Input: part model. Units: mm. Frame: model coordinates. A direction names the side the tool comes from. Give positions to 0.01 mm unless a question says otherwise; leave off trailing zeros. Order: outer loops, then holes, each group sorted by start corner. A loop starts at its lowest first (then second) coordinate and runs counter-clockwise, first axis right, second up. Notation, with made-up numbers: M -39,-38 L -8,-38 A36 cw -8,-1 Z; hole C -7,89.25 d1. An arc over 180 degrees is marked long. Use a Markdown table: item, result.
from build123d import *

# Parameters (mm, degrees)
BOSS_EXTRUDE1_DEPTH = 10
SKETCH2_R           = 1.5
CUT_EXTRUDE1_DEPTH  = 30


with BuildPart() as part:
    # Sketch1 → Boss-Extrude1 (new body)
    with BuildSketch(Plane.XY):
        with BuildLine():
            Line((-3, -2), (-14.8, -2))
            Line((-14.8, -2), (-15, -1.8))
            Line((-15, -1.8), (-15, -0.7))
            Line((-15, -0.7), (-14.8, -0.5))
            Line((-14.8, -0.5), (-4.866025404, -0.5))
            ThreePointArc((-4.866025404, -0.5), (-4.366025404, -0.366025404), (-4, 0))
            ThreePointArc((-4, 0), (-2.828427125, 2.828427125), (0, 4))
            Line((0, 4), (0, 2))
            ThreePointArc((0, 2), (-1.414213562, 1.414213562), (-2, 0))
            Line((-2, 0), (-2, -1))
            ThreePointArc((-2, -1), (-2.292893219, -1.707106781), (-3, -2))
        make_face()
    boss_extrude1 = extrude(amount=BOSS_EXTRUDE1_DEPTH)

    # Sketch2 → Cut-Extrude1 (cut)
    with BuildSketch(Plane(origin=(0, -0.5, 0), x_dir=(1, 0, 0), z_dir=(0, 1, 0))):
        with Locations(Location((-10, -5, 0), (0, 0, 180))):
            Circle(SKETCH2_R)
    cut_extrude1 = extrude(amount=-CUT_EXTRUDE1_DEPTH, mode=Mode.SUBTRACT)

    # Mirror1: Boss-Extrude1, Cut-Extrude1 across plane
    add(boss_extrude1.mirror(Plane(origin=(0, 2, 10), x_dir=(0, 0, 1), z_dir=(-1, 0, 0))))
    add(cut_extrude1.mirror(Plane(origin=(0, 2, 10), x_dir=(0, 0, 1), z_dir=(-1, 0, 0))), mode=Mode.SUBTRACT)


solid = part.part
1) Cut plane C-C on y = -1.45. Return loops of the section in (x, z), and give its area (3 significant figures).
Response values:
| item | result |
|---|---|
| outline | M -15,0 L -2.11,0 L -2.11,10 L -15,10 Z; M 2.11,0 L 15,0 L 15,10 L 2.11,10 Z; hole C -10,5 d3; hole C 10,5 d3 |
| area | 244 mm² |
2) Reachability of faces 5 (the face through (-15, -1, 5)), 6 (the face through (8.8, -0.5, 3.8)), 7 (the face through (15, -1, 5)), 8 (the face through (-2, -0.5, 4.9)), 9 (the face through (-8.8, -0.5, 3.8)) from +Z, -Z, +X, -X, +Y, -Y: full face, straight path, thin tool, end or side. Return the list, or none.
Response values:
| item | result |
|---|---|
| face 5 | +Z, -Z, -X, +Y, -Y |
| face 6 | +Z, -Z, +X, +Y |
| face 7 | +Z, -Z, +X, +Y, -Y |
| face 8 | +Z, -Z, -Y |
| face 9 | +Z, -Z, -X, +Y |
3) Mould query, pull axis Z, two halves, no side actions, for faces 1 (the face through (-1, 2, 0)), 2 (the face through (-8.5, -1.24, 5.07)), 3 (the face through (-1, 2, 10)), 4 (the face through (4.37, -0.37, 4.93)). Classes: released by +Z, released by -Z, zero draft, split by the parting line, or undercut.
Response values:
| item | result |
|---|---|
| face 1 | released by -Z |
| face 2 | undercut |
| face 3 | released by +Z |
| face 4 | zero draft |
4) Cut plane B-B on z = 5. Return loops of the section in (x, y).
Response values:
| item | result |
|---|---|
| outline | M -15,-1.8 L -14.8,-2 L -11.5,-2 L -11.5,-0.5 L -14.8,-0.5 L -15,-0.7 Z; M -8.5,-2 L -3,-2 A1 ccw -2,-1 L -2,0 A2 cw 2,0 L 2,-1 A1 ccw 3,-2 L 8.5,-2 L 8.5,-0.5 L 4.87,-0.5 A1 cw 4,0 A4 ccw -4,0 A1 cw -4.87,-0.5 L -8.5,-0.5 Z; M 11.5,-2 L 14.8,-2 L 15,-1.8 L 15,-0.7 L 14.8,-0.5 L 11.5,-0.5 Z |
5) First-contact query: pin 1 Ø1.5 at (y, z) = (3, 5) entering from -X; pin 2 Ø1.8 at (x, z) = (10, 5) entering from -Y; pin 3 Ø1.1 at (y, z) = (-0.5, 7.5) entering from +X. Flat tips, straight axial feed; report the tip coordinate or a pass-through.
Response values:
| item | result |
|---|---|
| pin 1 | stops at x = -3.31 |
| pin 2 | passes through |
| pin 3 | stops at x = 15 |
6) Cut plane D-D on z = 1. Return loops of the section in (x, y), and give its area (3 significant figures).
Response values:
| item | result |
|---|---|
| outline | M -15,-1.8 L -14.8,-2 L -3,-2 A1 ccw -2,-1 L -2,0 A2 cw 2,0 L 2,-1 A1 ccw 3,-2 L 14.8,-2 L 15,-1.8 L 15,-0.7 L 14.8,-0.5 L 4.87,-0.5 A1 cw 4,0 A4 ccw -4,0 A1 cw -4.87,-0.5 L -14.8,-0.5 L -15,-0.7 Z |
| area | 59.6 mm² |
7) Cut plane A-A on x = 10. Return loops of the section in (y, z).
Response values:
| item | result |
|---|---|
| outline | M -2,0 L -0.5,0 L -0.5,3.5 L -2,3.5 Z; M -2,6.5 L -0.5,6.5 L -0.5,10 L -2,10 Z |
8) Material intervals for line 1 (Z direction, x = 10, y = -1.05); line 2 (X direction, y = 1.7, z = 5.75); line 3 (Y direction, x = 0, z = 8.25), sorted ascending. Write a range as from..to.
Response values:
| item | result |
|---|---|
| line 1 | z = 0..3.5, 6.5..10 |
| line 2 | x = -3.62..-1.05, 1.05..3.62 |
| line 3 | y = 2..4 |
